The listing builds one solid part. Answer for the finished solid, in the listing's coordinates (mm). Coordinates: 2 decimals unless noted, no trailing zeros. Write each loop counter-clockwise with the first axis right and the second up, starting at its lowest first coordinate (ties: lowest second). Pieces come first, ordered by that corner, then holes.
Autodesk Inventor part; units mm, degrees
ref_plane "YZ Plane" through (0, 0, 0) normal (1, 0, 0) x (0, 1, 0)
ref_plane "XY Plane" through (0, 0, 0) normal (0, 0, 1) x (1, 0, 0)
ref_plane "Work Plane1" through (0, 193, 0) normal (0, 1, 0) x (-1, 0, 0)
sketch "Sketch1" plane through (0, 193, 0) normal (0, 1, 0) x (-1, 0, 0)
  line L0 (0, -83.592) -> (0, 13.932) construction
  line L1 (438.46, 0) -> (-674.96, 0) construction
  line L2 (279.4, -15.35) -> (278.2, -22.85)
  line L3 (278.2, -22.85) -> (65, -47.86)
  line L4 (65, -47.86) -> (-358.9, -51.36)
  line L5 (-358.9, -51.36) -> (-515.9, -69.66)
  line L6 (-515.9, -69.66) -> (-515.9, -47.66)
  line L7 (-515.9, -47.66) -> (-359.9, -15.93)
  line L8 (-359.9, -15.93) -> (279.4, -15.35)
  point P0 (0, 0)
  dimension "d1" = 22.85
  dimension "d2" = 47.86
  dimension "d3" = 15.35
  dimension "d4" = 279.4
  dimension "d5" = 278.2
  dimension "d6" = 65
  dimension "d7" = 51.36
  dimension "d8" = 69.66
  dimension "d9" = 47.66
  dimension "d10" = 15.93
  dimension "d11" = 515.9
  dimension "d12" = 515.9
  dimension "d13" = 358.9
  dimension "d14" = 359.9
extrude "Extrusion1" add sketch "Sketch1" along normal mid plane 28
properties part number "Friend_sideskirt_collision"
Q1. The part is cut by section B-B, the plane x = 320. Write down the section's boundary in (y, z).
Answers below:
outline: (179, -51.04) - (207, -51.04) - (207, -15.89) - (179, -15.89) - close
Q2. The part is cut by section C-C, the plane z = -33. Write down the section's boundary in (x, y), then the cut area to 3 significant figures.
Answers below:
outline: (-191.68, 179) - (443.82, 179) - (443.82, 207) - (-191.68, 207) - close
area: 17,800 mm2
Q3. Given pin 1 (10 mm diameter, centred on x = 402.5, y = 192, fed in from -Z); pin 2 (1.5 mm diameter, centred on x = 118.5, y = 197, fed in from +Z); pin 3 (2 mm diameter, centred on x = 148.5, y = 203.5, fed in from -Z), each flat-ended and moving along its own axis, determine where each tip first touches the part or whether it passes through.
Answers below:
pin 1: stops at z = -57.02
pin 2: stops at z = -15.71
pin 3: stops at z = -49.63
Q4. The part is cut by section A-A, the plane y = 189. Write down the section's boundary in (x, z), then the cut area to 3 significant figures.
Answers below:
outline: (-279.4, -15.35) - (-278.2, -22.85) - (-65, -47.86) - (358.9, -51.36) - (515.9, -69.66) - (515.9, -47.66) - (359.9, -15.93) - close
area: 23,100 mm2
Q5. Find the intervals of material crossed by probe 1 along Z at (x, y) = (416.5, 195.5); probe 2 along Z at (x, y) = (69.5, 205.25), in increasing order.
Answers below:
probe 1: z = -58.07 to -27.44
probe 2: z = -48.97 to -15.67
